Can you work these out from the model? Positions are in its coordinate system, mm. A direction names the side the tool comes from. Give positions to 0.01 mm unless a question says otherwise; leave off trailing zeros. Order: outer loops, then holes, each group sorted by start corner. A loop starts at its lowest first (then second) coordinate and runs counter-clockwise, first axis right, second up.
```python
from build123d import *

# Parameters (mm, degrees)
ESQUISSE1_W      = 55
ESQUISSE1_H      = 33
ESQUISSE1_R      = 1.5
EXTRUSION1_DEPTH = 3
ESQUISSE2_W      = 7.634201779
ESQUISSE2_H      = 7.63420178
ESQUISSE2_W_2    = 5.337752956
ESQUISSE2_H_2    = 14.027301674
ESQUISSE2_W_3    = 5.224355128
ESQUISSE2_H_3    = 5.224355128
EXTRUSION2_DEPTH = 18
ESQUISSE3_R      = 3.279080348
EXTRUSION3_DEPTH = 12
ESQUISSE4_W      = 4
ESQUISSE4_H      = 19.646099489
EXTRUSION4_DEPTH = 23


with BuildPart() as part:
    # Esquisse1 → Extrusion1 (new body)
    with BuildSketch(Plane(origin=(0, 0, 0), x_dir=(1, 0, 0), z_dir=(0, 1, 0))):
        with Locations((27.5, 16.5)):
            Rectangle(ESQUISSE1_W, ESQUISSE1_H)
        with Locations((5, 28)):
            Circle(ESQUISSE1_R, mode=Mode.SUBTRACT)
        with Locations((50, 28)):
            Circle(ESQUISSE1_R, mode=Mode.SUBTRACT)
        with Locations((50, 5)):
            Circle(ESQUISSE1_R, mode=Mode.SUBTRACT)
        with Locations((5, 5)):
            Circle(ESQUISSE1_R, mode=Mode.SUBTRACT)
    extrude(amount=EXTRUSION1_DEPTH)

    # Esquisse2 → Extrusion2 (add)
    with BuildSketch(Plane(origin=(0, 3, 0), x_dir=(1, 0, 0), z_dir=(0, 1, 0))):
        with Locations((33.593446124, 26.205676479)):
            Rectangle(ESQUISSE2_W, ESQUISSE2_H)
        with Locations((51.457386868, 17.801055276)):
            Rectangle(ESQUISSE2_W_2, ESQUISSE2_H_2)
        with Locations((11.46939236, 25.577155504)):
            Rectangle(ESQUISSE2_W_3, ESQUISSE2_H_3)
        with Locations((22.552159567, 25.577155504)):
            Rectangle(ESQUISSE2_W_3, ESQUISSE2_H_3)
    extrude(amount=EXTRUSION2_DEPTH)

    # Esquisse3 → Extrusion3 (add)
    with BuildSketch(Plane(origin=(0, 3, 0), x_dir=(1, 0, 0), z_dir=(0, 1, 0))):
        with Locations((11.5, 8.756763264)):
            Circle(ESQUISSE3_R)
        with Locations((19.5, 8.756763264)):
            Circle(ESQUISSE3_R)
        with Locations((27.5, 8.756763264)):
            Circle(ESQUISSE3_R)
        with Locations((35.5, 8.756763264)):
            Circle(ESQUISSE3_R)
    extrude(amount=EXTRUSION3_DEPTH)

    # Esquisse4 → Extrusion4 (add)
    with BuildSketch(Plane(origin=(0, 3, 0), x_dir=(1, 0, 0), z_dir=(0, 1, 0))):
        with Locations((43.737455539, 15.895279312)):
            Rectangle(ESQUISSE4_W, ESQUISSE4_H)
    extrude(amount=EXTRUSION4_DEPTH)


solid = part.part
```
1) Suppose I cut it at D-D (y = 6.75). Give the number of separate pieces and of enclosed holes in the cut face, and give its area (3 significant figures).
2) Suppose I cut it at B-B (x = 50). Please give me the cut outline in (y, z).
3) Which directions (+Z, -Z, +X, -X, +Y, -Y) give clear straight access to the entire face, cutting with the end or side of a thin tool? Please do faces 4 (the face through (51, 21, -18)), 5 (the face through (51, 12, -10.787)), 6 (the face through (23, 12, -22.965)).
4) Suppose I cut it at C-C (z = -15). Please give me the cut outline in (x, y), and give its area (3 significant figures).
5) If I drill on line 1 (X direction, y = 12.75, z = -25.5); line 2 (X direction, y = 1.65, z = -28); line 3 (Z direction, x = 50, y = 1.3), over which ranges is the centre line in solid material (lowest first)?
6) I'm going to push flat-ended pins straight in: pin 1 Ø2.5 at (y, z) = (8, -24.5) entering from +X; pin 2 Ø1.2 at (x, y) = (43.5, 19.5) entering from -Z; pin 3 Ø5 at (x, z) = (35.5, -7.5) entering from +Y. Where does each tip first touch, or does it pass through?
7) We'd pull the mould along Z, two halves only. Please class faces 1 (the face through (14.53, 8.92, -7.5)), 2 (the face through (51, 12, -24.815)), 3 (the face through (27, 15, -9)): +Z half, -Z half, draft (parallel to the pull), parting line (faces both ways), or undercut.
8) Suppose I cut it at A-A (y = 18.75). Please give me the cut outline in (x, z), and give its area (3 significant figures).
Results:
1. separate pieces: 9
1. enclosed holes: 0
1. area: 401 mm2
2. outline: (0, -33) - (3, -33) - (3, -29.5) - (0, -29.5) - close; (0, -26.5) - (3, -26.5) - (3, -24.81) - (21, -24.81) - (21, -10.79) - (3, -10.79) - (3, -6.5) - (0, -6.5) - close; (0, -3.5) - (3, -3.5) - (3, 0) - (0, 0) - close
3. face 4: +Z, -Z, +X, +Y
3. face 5: +Z, +X, +Y
3. face 6: -X, +Y
4. outline: (0, 0) - (55, 0) - (55, 3) - (54.13, 3) - (54.13, 21) - (48.79, 21) - (48.79, 3) - (45.74, 3) - (45.74, 26) - (41.74, 26) - (41.74, 3) - (0, 3) - close
4. area: 353 mm2
5. line 1: x = 8.86 to 14.08, 19.94 to 25.16, 29.78 to 37.41, 41.74 to 45.74
5. line 2: x = 0 to 3.5, 6.5 to 48.5, 51.5 to 55
5. line 3: z = -33 to -29.5, -26.5 to -6.5, -3.5 to 0
6. pin 1: stops at x = 54.13
6. pin 2: stops at z = -25.72
6. pin 3: stops at y = 15
7. face 1: undercut
7. face 2: -Z half
7. face 3: draft
8. outline: (8.86, -28.19) - (14.08, -28.19) - (14.08, -22.96) - (8.86, -22.96) - close; (19.94, -28.19) - (25.16, -28.19) - (25.16, -22.96) - (19.94, -22.96) - close; (29.78, -30.02) - (37.41, -30.02) - (37.41, -22.39) - (29.78, -22.39) - close; (41.74, -25.72) - (45.74, -25.72) - (45.74, -6.07) - (41.74, -6.07) - close; (48.79, -24.81) - (54.13, -24.81) - (54.13, -10.79) - (48.79, -10.79) - close
8. area: 266 mm2
